Autodesk Inventor part; units mm, degrees
ref_plane "YZ Plane" through (0, 0, 0) normal (1, 0, 0) x (0, 1, 0)
ref_plane "XY Plane" through (0, 0, 0) normal (0, 0, 1) x (1, 0, 0)
sketch "Sketch1" plane through (0, 0, 0) normal (0, 0, 1) x (1, 0, 0)
  line L0 (195.2625, 4.445) -> (195.2625, -4.445)
  line L1 (-7.9375, -7.62) -> (-7.9375, 7.62)
  circle A0 centre (0, 0) radius 0.4079
  arc A1 (195.2625, 4.445) -> (192.0875, 7.62) centre (192.0875, 4.445) ccw
  arc A2 (192.0875, -7.62) -> (195.2625, -4.445) centre (192.0875, -4.445) ccw
  line L2 (111.9187, 25.4) -> (142.0813, 25.4)
  line L3 (142.0813, -25.4) -> (111.9187, -25.4)
  line L4 (127, 42.8625) -> (127, -39.6875) construction
  line L5 (127, 19.8437) -> (127, 19.8437)
  line L6 (133.35, 13.4937) -> (133.35, -13.4937)
  line L7 (127, -19.8437) -> (127, -19.8437)
  line L8 (120.65, -13.4937) -> (120.65, 13.4938)
  arc A3 (127, 19.8437) -> (120.65, 13.4938) centre (127, 13.4937) ccw
  arc A4 (133.35, 13.4937) -> (127, 19.8437) centre (127, 13.4937) ccw
  arc A5 (127, -19.8437) -> (133.35, -13.4937) centre (127, -13.4937) ccw
  arc A6 (120.65, -13.4937) -> (127, -19.8437) centre (127, -13.4937) ccw
  line L9 (-7.9375, 7.62) -> (111.9187, 7.62)
  line L10 (142.0813, 7.62) -> (192.0875, 7.62)
  line L11 (192.0875, -7.62) -> (142.0813, -7.62)
  line L12 (111.9187, -7.62) -> (-7.9375, -7.62)
  line L13 (111.9187, -25.4) -> (111.9187, -7.62)
  line L14 (111.9187, 7.62) -> (111.9187, 25.4)
  line L15 (142.0813, 25.4) -> (142.0813, 7.62)
  line L16 (142.0813, -7.62) -> (142.0813, -25.4)
  point P0 (-7.9375, 0)
  point P1 (127, 25.4)
  point P2 (111.9187, 0)
  point P3 (120.65, 0)
  dimension "d0" = 15.24
  dimension "d1" = 203.2
  dimension "d2" = 3.175
  dimension "d3" = 127
  dimension "d4" = 6.35
  dimension "d43" = 25.4
  dimension "d44" = 25.4
extrude "Extrusion1" add sketch "Sketch1" along normal blind 6.35
ref_plane "Work Plane3" through (127, 7.62, 0) normal (1, 0, 0) x (0, 0, -1)
fillet "Fillet1" radius 6.35 8 edges at (142.0813, -25.4, 3.175) (111.9187, -25.4, 3.175) (142.0813, 25.4, 3.175) (111.9187, 25.4, 3.175) (142.0813, -7.62, 3.175) (111.9187, -7.62, 3.175) (111.9187, 7.62, 3.175) (142.0813, 7.62, 3.175)
sketch "Sketch10" plane through (0, 0, 6.35) normal (0, 0, 1) x (1, 0, 0)
  line L0 (144.0488, 3.81) -> (184.4165, 3.81)
  line L1 (187.5915, 0.635) -> (187.5915, -0.635)
  line L2 (184.4165, -3.81) -> (144.0488, -3.81)
  line L3 (140.8738, -0.635) -> (140.8738, 0.635)
  arc A0 (111.9187, -19.05) -> (118.2688, -25.4) centre (118.2688, -19.05) ccw
  line L4 (135.7313, -25.4) -> (118.2688, -25.4)
  arc A1 (135.7313, -25.4) -> (142.0813, -19.05) centre (135.7313, -19.05) ccw
  arc A2 (148.4313, -7.62) -> (142.0813, -13.97) centre (148.4313, -13.97) ccw
  line L5 (192.0875, -7.62) -> (148.4313, -7.62)
  arc A3 (192.0875, -7.62) -> (195.2625, -4.445) centre (192.0875, -4.445) ccw
  line L6 (195.2625, 4.445) -> (195.2625, -4.445)
  arc A4 (195.2625, 4.445) -> (192.0875, 7.62) centre (192.0875, 4.445) ccw
  line L7 (148.4313, 7.62) -> (192.0875, 7.62)
  arc A5 (142.0813, 13.97) -> (148.4313, 7.62) centre (148.4313, 13.97) ccw
  arc A6 (142.0813, 19.05) -> (135.7313, 25.4) centre (135.7313, 19.05) ccw
  line L8 (118.2687, 25.4) -> (135.7313, 25.4)
  arc A7 (118.2687, 25.4) -> (111.9187, 19.05) centre (118.2687, 19.05) ccw
  arc A8 (105.5687, 7.62) -> (111.9187, 13.97) centre (105.5687, 13.97) ccw
  line L9 (-7.9375, 7.62) -> (105.5687, 7.62)
  line L10 (-7.9375, -7.62) -> (-7.9375, 7.62)
  line L11 (105.5687, -7.62) -> (-7.9375, -7.62)
  arc A9 (111.9187, -13.97) -> (105.5687, -7.62) centre (105.5687, -13.97) ccw
  arc A10 (133.35, 13.4937) -> (120.65, 13.4938) centre (127, 13.4937) ccw
  line L12 (133.35, 13.4937) -> (133.35, -13.4937)
  arc A11 (120.65, -13.4937) -> (133.35, -13.4937) centre (127, -13.4937) ccw
  line L13 (120.65, -13.4937) -> (120.65, 13.4938)
  circle A12 centre (0, 0) radius 0.4079
  line L14 (-7.9375, 7.62) -> (82.3369, 7.62)
  line L15 (82.3369, 7.62) -> (89.9679, 7.62)
  line L16 (195.2625, 4.445) -> (195.2625, -4.445)
  arc A13 (144.0488, 3.81) -> (140.8738, 0.635) centre (144.0488, 0.635) ccw
  arc A14 (140.8738, -0.635) -> (144.0488, -3.81) centre (144.0488, -0.635) ccw
  arc A15 (187.5915, 0.635) -> (184.4165, 3.81) centre (184.4165, 0.635) ccw
  arc A16 (184.4165, -3.81) -> (187.5915, -0.635) centre (184.4165, -0.635) ccw
  line L17 (-7.9375, 0) -> (195.2625, 0)
  line L18 (-7.9375, -7.62) -> (82.3369, -7.62)
  line L19 (82.3369, -7.62) -> (89.9679, -7.62)
  line L20 (142.0813, -13.97) -> (142.0813, -19.05)
  line L21 (142.0813, 19.05) -> (142.0813, 13.97)
  line L22 (111.9187, 13.97) -> (111.9187, 19.05)
  line L23 (111.9187, -19.05) -> (111.9187, -13.97)
  point P0 (187.5915, 0)
  point P1 (140.8738, 0)
  dimension "d22" = 3.175
  dimension "d23" = 7.62
  dimension "d24" = 3.175
  dimension "d25" = 7.62
  dimension "d26" = 7.62
extrude "Extrusion7" cut sketch "Sketch10" against normal through all contours L0 A15 L1 L17 L3 A13 | L17 L1 A16 L2 A14 L3
sketch "Sketch7" plane through (0, 0, 0) normal (0, 1, 0) x (-1, 0, 0)
  line L0 (7.9375, 0) -> (7.9375, -5)
  line L1 (7.9375, 0) -> (-19.05, 0)
  line L2 (-111.9187, 0) -> (7.9375, 0)
  line L3 (7.9375, 0) -> (1.5875, 0)
  line L4 (1.5875, 0) -> (1.5875, -5)
  line L5 (7.9375, -5) -> (7.9375, 0)
  arc A0 (1.5875, -5) -> (7.9375, -5) centre (4.7625, -5) ccw
  circle A1 centre (4.7625, -5) radius 1.5875
  line L6 (1.5875, -5) -> (3.175, -5)
  line L7 (6.35, -5) -> (7.9375, -5)
  line L8 (7.9375, 0) -> (-111.9187, 0)
  point P0 (0, 0)
  point P1 (-89.9679, 0)
  dimension "d35" = 6.35
  dimension "d40" = 5
  dimension "d41" = 3.175
  dimension "d42" = 3.175
extrude "Extrusion9" add sketch "Sketch7" along normal mid plane 15.24 contours L0 L7 A1 L6 L4 L1 | A0 L6 A1 L7
sketch "Sketch12" plane through (0, 0, 0) normal (0, 1, 0) x (-1, 0, 0)
  line L0 (1.5875, 0) -> (7.9375, 0)
  arc A0 (1.5875, -5) -> (7.9375, -5) centre (4.7625, -5) ccw
  arc A1 (1.5875, -5) -> (7.9375, -5) centre (4.7625, -5) ccw
  line L1 (7.9375, 6.35) -> (7.9375, -5)
  line L2 (1.5875, -5) -> (1.5875, 0)
  point P0 (0, 0)
extrude "Extrusion11" cut sketch "Sketch12" against normal mid plane 7.62
chamfer "Chamfer1" distance 2.54 angle 45 1 edges at (-7.9375, 0, 6.35)
properties part number "Scottish Yoke" material "Steel, High Strength Low Alloy"
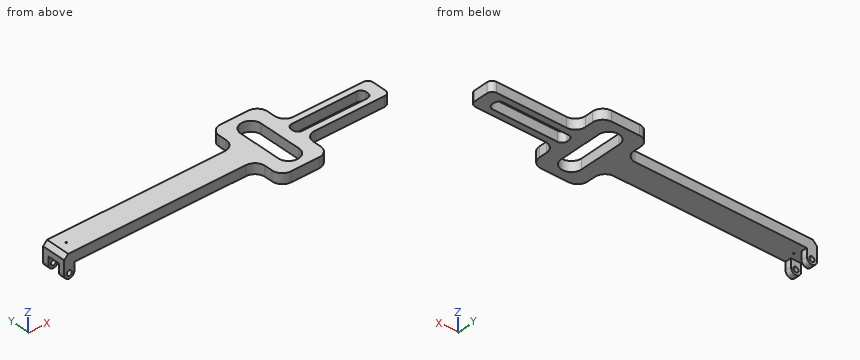
Input: part model. Units: mm. Frame: model coordinates. Coordinates: 2 decimals unless noted, no trailing zeros. Loops run counter-clockwise (first coordinate to the right, second up) from the corner with the lowest first, then second, coordinate; pieces in that order, holes last. Notation, with made-up numbers: M 49,43.25 L 100,43.25 A13 ccw 100,61.25 Z; hole C -31,-32.75 d6. An arc over 180 degrees is marked long. Use a Markdown table: item, result. Add a question column.
1) Section C-C, the plane x = 32.5. Return the cut outline in (y, z), plus the area to 3 significant figures.
2) Pin query (flat end, axial travel): P1, Ø7.5, axis at x = 62, z = -3, coming from the +Y side; P2, Ø1.5, axis at y = 5, z = -5, coming from the +X side; P3, Ø5, axis at x = 174, z = 2.5, coming from the -Y side. Return the tip coordinate at first contact, or that it passes through.
3) Section A-A, the plane x = 127. Return the cut outline in (y, z).
4) Line query: L1, parallel to Y at x = 152.5, z = 3; L2, parallel to Y at x = 0, z = 4; L3, parallel to Z at x = 115.5, y = -20.5. Output: solid intervals per line, ascending. Write a range as from..to.
5) Section B-B, the plane y = 17. Return the cut outline in (x, z).
Answer below:
| question | item | result |
|---|---|---|
| 1 | outline | M -7.62,0 L 7.62,0 L 7.62,6.35 L -7.62,6.35 Z |
| 1 | area | 96.8 mm2 |
| 2 | P1 | y = 7.62 |
| 2 | P2 | x = -1.59 |
| 2 | P3 | y = -7.62 |
| 3 | outline | M -25.4,0 L -19.84,0 L -19.84,6.35 L -25.4,6.35 Z; M 19.84,0 L 25.4,0 L 25.4,6.35 L 19.84,6.35 Z |
| 4 | L1 | -7.62..-3.81, 3.81..7.62 |
| 4 | L2 | -7.62..-0.41, 0.41..7.62 |
| 4 | L3 | 0..6.35 |
| 5 | outline | M 111.92,0 L 121.71,0 L 121.71,6.35 L 111.92,6.35 Z; M 132.29,0 L 142.08,0 L 142.08,6.35 L 132.29,6.35 Z |
